Can you work these out from the drawing? Everything is in mm from the part's minimum corner. A direction names the side the tool comes from. Round coordinates to 2 decimals unless told otherwise and drop trailing zeros. Loops run counter-clockwise (first coordinate to the right, second up) from the corner with the lowest first, then second, coordinate; pieces in that order, holes last. Notation, with made-up numbers: (20.5, 33) - (68.5, 33) arc R25 cw to (68.5, 67) - close; hole circle Ø3 at (28, 52). An arc over 180 degrees is marked (long way). Answer as a JSON object with one key per item and string values. Group by question number.
1) Will this pin go through, and if not, where does the flat tip stop? P1, Ø2, axis at x = 42, z = 98.5, coming from the +Y side (3 decimals).
2) Which directions (+Z, -Z, +X, -X, +Y, -Y) give clear straight access to the entire face, cutting with the end or side of a thin tool? Please do the marked faces 1 and 2.
3) I want a section at C-C, the plane z = 35. Please give me the cut outline in (x, y) (3 decimals).
4) I want a section at B-B, the plane x = 47. Please give me the cut outline in (y, z) (3 decimals).
5) I want a section at A-A, the plane y = 18.75. Please give me the cut outline in (x, z) (3 decimals), then the cut area to 3 significant figures.
6) If we mould it in two halves opening along X, with no side actions, what happens to the marked faces 3, 4 and 5? For each: pulls with the +X half, pulls with the -X half, needs draft (parallel to the pull), parting line crosses it, or undercut.
7) If I drill on line 1 along Z through (x, y) = (13.5, 18) (3 decimals); line 2 along X through (y, z) = (17.25, 80) (3 decimals); line 3 along Y through (x, z) = (13.5, 102) (3 decimals), over which ranges is the centre line in solid material (lowest first)? Write a range as [from, to].
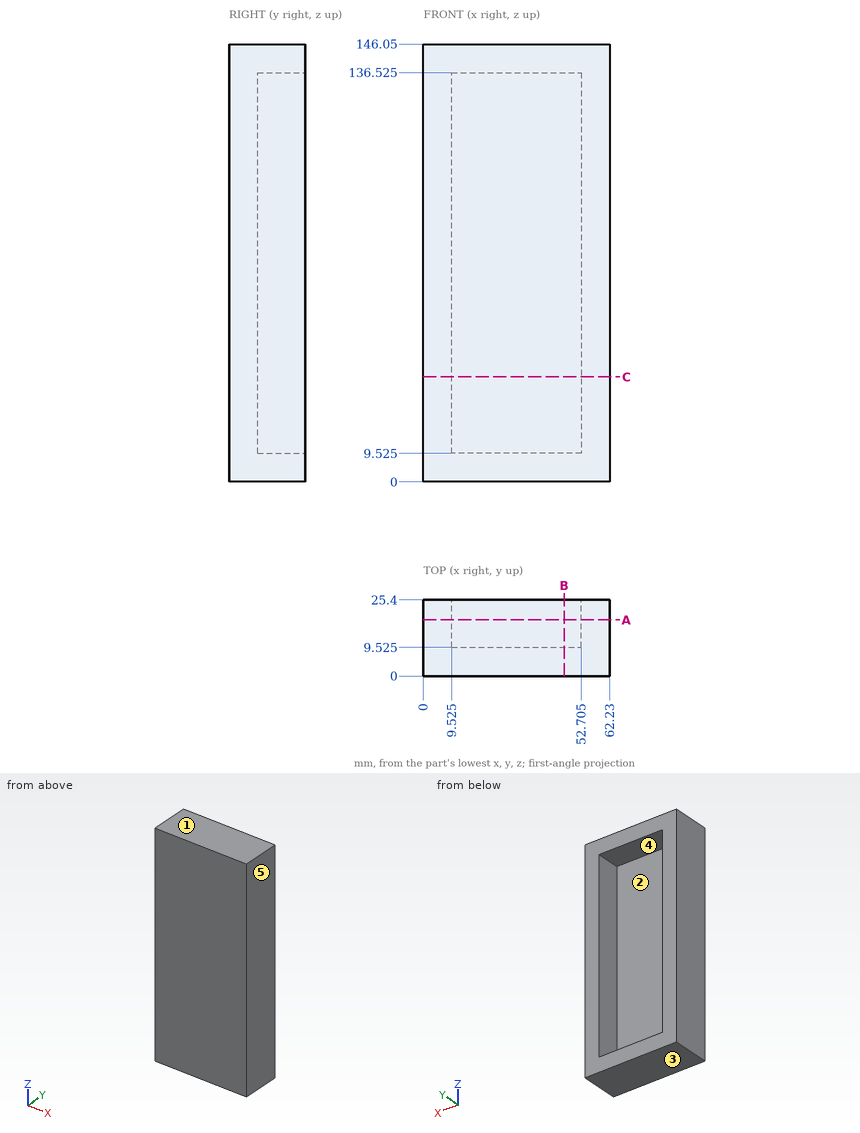
Outcome:
{
 "1": {"P1": "y = 9.525"},
 "2": {"face 1": "+Z, +X, -X, +Y, -Y", "face 2": "+Y"},
 "3": {"outline": "(0, 0) - (62.23, 0) - (62.23, 25.4) - (52.705, 25.4) - (52.705, 9.525) - (9.525, 9.525) - (9.525, 25.4) - (0, 25.4) - close"},
 "4": {"outline": "(0, 0) - (25.4, 0) - (25.4, 9.525) - (9.525, 9.525) - (9.525, 136.525) - (25.4, 136.525) - (25.4, 146.05) - (0, 146.05) - close"},
 "5": {"outline": "(0, 0) - (62.23, 0) - (62.23, 146.05) - (0, 146.05) - close; hole (9.525, 9.525) - (52.705, 9.525) - (52.705, 136.525) - (9.525, 136.525) - close", "area": "3,600 mm^2"},
 "6": {"face 3": "needs draft", "face 4": "undercut", "face 5": "pulls with the +X half"},
 "7": {"line 1": "[0, 9.525], [136.525, 146.05]", "line 2": "[0, 9.525], [52.705, 62.23]", "line 3": "[0, 9.525]"}
}
